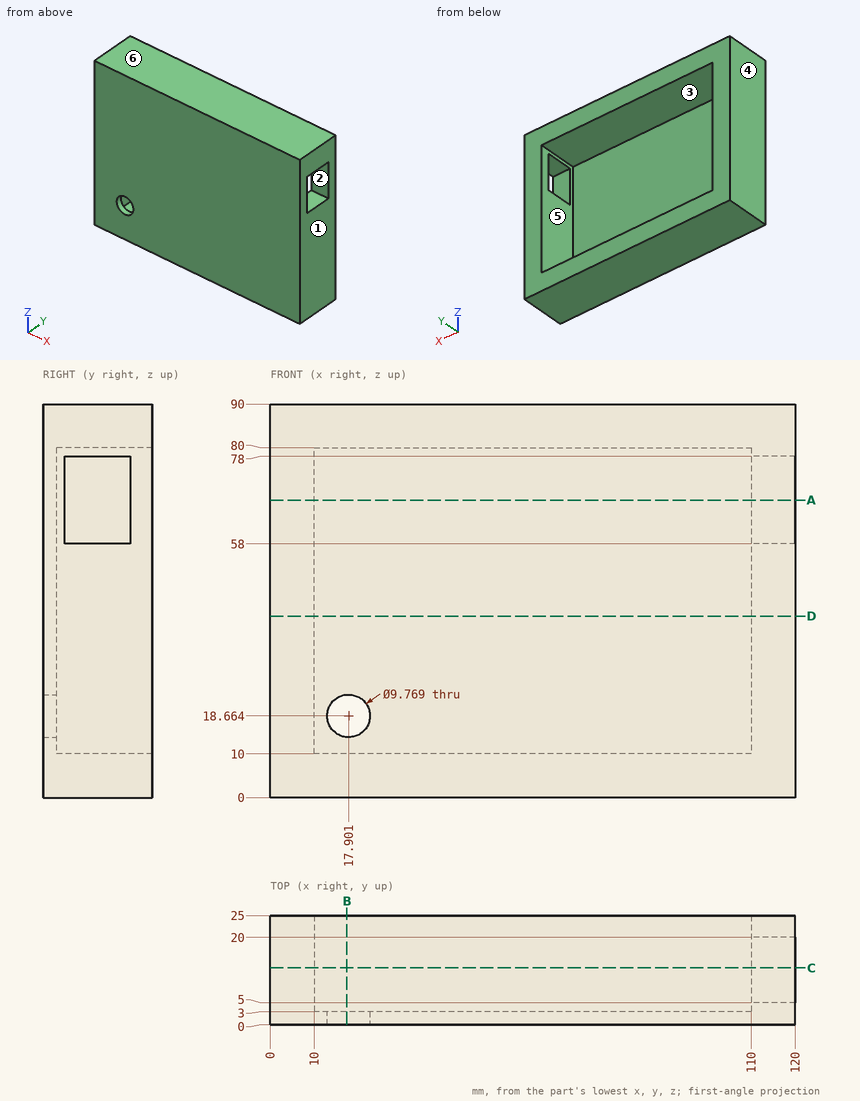
Check sheet for the drawn part. Datum: minimum x, y, z corner. Units: mm. A direction names the side the tool comes from. Coordinates: 2 decimals unless noted, no trailing zeros. Order: outer loops, then holes, each group sorted by start corner. A loop starts at its lowest first (then second) coordinate and runs counter-clockwise, first axis right, second up. Notation, with made-up numbers: (-19, 16.25) - (35, 16.25) arc R27 cw to (35, 45.25) - close; hole circle Ø2 at (4, 29.25). An arc over 180 degrees is marked (long way). Return JSON: item names as keys, results as strings.
(1) Section check B-B, the plane x = 17.5. Record the cut outline in (y, z), and give its area (3 significant figures).
Filled sheet:
{"outline": "(0, 0) - (25, 0) - (25, 10) - (3, 10) - (3, 13.8) - (0, 13.8) - close; (0, 23.53) - (3, 23.53) - (3, 80) - (25, 80) - (25, 90) - (0, 90) - close", "area": "681 mm^2"}
(2) Access from +Z, -Z, +X, -X, +Y, -Y to the whole of each face (thin tool, end or side, straight path). Record for the marked faces 1, 2 and 3.
Filled sheet:
{"face 1": "+Z, -Z, +X, +Y, -Y", "face 2": "+X", "face 3": "+Y"}
(3) Thickness scan on line 1 along X through (y, z) = (3.5, 70); line 2 along Z through (x, y) = (37, 15); line 3 along X through (y, z) = (17.5, 72). Record the ranges inside material, lowest first.
Filled sheet:
{"line 1": "x = 0 to 10, 110 to 120", "line 2": "z = 0 to 10, 80 to 90", "line 3": "x = 0 to 10"}
(4) Section check D-D, the plane z = 41.5. Record the cut outline in (x, y), and give its area (3 significant figures).
Filled sheet:
{"outline": "(0, 0) - (120, 0) - (120, 25) - (110, 25) - (110, 3) - (10, 3) - (10, 25) - (0, 25) - close", "area": "800 mm^2"}
(5) Section check C-C, the plane y = 13. Record the cut outline in (x, z), and give its area (3 significant figures).
Filled sheet:
{"outline": "(0, 0) - (120, 0) - (120, 58) - (110, 58) - (110, 10) - (10, 10) - (10, 80) - (110, 80) - (110, 78) - (120, 78) - (120, 90) - (0, 90) - close", "area": "3,600 mm^2"}
(6) Section check A-A, the plane z = 68. Record the cut outline in (x, y).
Filled sheet:
{"outline": "(0, 0) - (120, 0) - (120, 5) - (110, 5) - (110, 3) - (10, 3) - (10, 25) - (0, 25) - close; (110, 20) - (120, 20) - (120, 25) - (110, 25) - close"}
(7) Go/stop test with a flat-tipped pin: pin 1 (3 mm diameter, centred on x = 45, z = 36, fed in from +Y). Record where the tip stops, or that it passes through.
Filled sheet:
{"pin 1": "stops at y = 3"}
(8) Mould release check, pull along Z, two halves, no side actions. Record for the marked faces 4, 5 and 6: pulls with the +Z half, pulls with the -Z half, needs draft (parallel to the pull), parting line crosses it, or undercut.
Filled sheet:
{"face 4": "needs draft", "face 5": "undercut", "face 6": "pulls with the +Z half"}
